from build123d import *

# Parameters (mm, degrees)
ESQUISSE1_W             = 168
ESQUISSE1_H             = 78
BOSS_EXTRU_1_DEPTH      = 3
CONG_1_R                = 3
ESQUISSE2_R             = 1.5
ENL_V_MAT_EXTRU_1_DEPTH = 186.248481775


with BuildPart() as part:
    # Esquisse1 → Boss.-Extru.1 (new body)
    with BuildSketch(Plane.XY):
        with Locations((84, 39)):
            Rectangle(ESQUISSE1_W, ESQUISSE1_H)
    extrude(amount=BOSS_EXTRU_1_DEPTH)

    # Congé1
    cong_1_edges = [part.edges().sort_by_distance(p)[0] for p in [
        (0, 78, 1.5),
        (168, 78, 1.5),
        (168, 0, 1.5),
        (0, 0, 1.5),
    ]]
    fillet(cong_1_edges, radius=CONG_1_R)

    # Esquisse2 → Enlèv. mat.-Extru.1 (cut, through all)
    with BuildSketch(Plane.XY.offset(3)):
        with Locations((84, 68)):
            Circle(ESQUISSE2_R)
    extrude(amount=-ENL_V_MAT_EXTRU_1_DEPTH, mode=Mode.SUBTRACT)


solid = part.part
Part model, mm, in its own coordinate system. Coordinates: 2 decimals unless noted, no trailing zeros. Loops run counter-clockwise (first coordinate to the right, second up) from the corner with the lowest first, then second, coordinate; pieces in that order, holes last. Notation, with made-up numbers: (76, 14.5) -> (103, 14.5) arc R30 cw to (103, 48.5) -> close; hole circle Ø6 at (32, 57). An arc over 180 degrees is marked (long way). Use a Markdown table: item, result. Add a question column.
Item 1: Band-saw the part on A-A on y = 68. Write the cut outline in (x, z), plus the area to 3 significant figures.
Item 2: Probe probe 1 along X at (y, z) = (68, 2.25); probe 2 along Y at (x, z) = (84, 2.4). List the from-to ranges inside material, lowest first.
Item 3: Pull direction X, two halves, no side cores. Call faces 1 (the flat face through (83, 0, 1)), 2 (the cylindrical face through (84.806, 69.265, 1.521)), 3 (the cylindrical face through (167.1, 0.86, 1.52)): +X half, -X half, draft (parallel to the pull), parting line (faces both ways), or undercut.
Item 4: Band-saw the part on B-B on x = 84. Write the cut outline in (y, z).
Geometry says:
| question | item | result |
|---|---|---|
| 1 | outline | (0, 0) -> (82.5, 0) -> (82.5, 3) -> (0, 3) -> close; (85.5, 0) -> (168, 0) -> (168, 3) -> (85.5, 3) -> close |
| 1 | area | 495 mm² |
| 2 | probe 1 | 0 to 82.5, 85.5 to 168 |
| 2 | probe 2 | 0 to 66.5, 69.5 to 78 |
| 3 | face 1 | draft |
| 3 | face 2 | undercut |
| 3 | face 3 | +X half |
| 4 | outline | (0, 0) -> (66.5, 0) -> (66.5, 3) -> (0, 3) -> close; (69.5, 0) -> (78, 0) -> (78, 3) -> (69.5, 3) -> close |
